Could you check a few things on this model? Use its own coordinates, in mm. Face numbers are marked on the shaded views. A direction names the side the tool comes from. Give positions to 0.01 mm unless a question says otherwise; leave off trailing zeros. Loops run counter-clockwise (first coordinate to the right, second up) from the corner with the lowest first, then second, coordinate; pieces in that order, holes last. Notation, with made-up numbers: (67, -7.75) -> (108, -7.75) arc R14 cw to (108, 8.25) -> close; hole circle Ø11 at (70.25, 79). An arc over 180 degrees is marked (long way). Write item = value, one per line. Start each with the question number.
1) I want a section at C-C (y = 8). Count the separate pieces of the cut face and the enclosed holes in it, and give its area (3 significant figures).
2) If we mould it in two halves opening along Z, with no side actions, what happens to the marked faces 1, 2 and 3? For each: +Z half, -Z half, draft (parallel to the pull), parting line (faces both ways), or undercut.
3) I want a section at D-D (z = -67). List the corners of the cut face in (x, y) for me, and give its area (3 significant figures).
4) I want a section at B-B (z = -5). List the corners of the cut face in (x, y) for me, and give its area (3 significant figures).
5) I'm going to push a flat-ended pin straight in: pin 1 Ø3.5 at (x, z) = (-5, -50.5) entering from +Y. Where does the tip first touch, or does it pass through?
6) On a 3-axis mill with a long thin cutter (end or side, diameter ignored), from which of +Z, -Z, +X, -X, +Y, -Y can I reach the whole of each face in a straight line? I mean the marked faces 4 and 5. Say none if no direction works.
7) I need wall thicknesses on probe 1 along Z at (x, y) = (-5.5, 1.7); probe 2 along Z at (x, y) = (-2.25, 12); probe 3 along Y at (x, z) = (2.75, -76). Which ranges of each line are inside material? Lowest first, please. Write a range as from..to.
8) I want a section at A-A (x = -5.5). List the corners of the cut face in (y, z) for me.
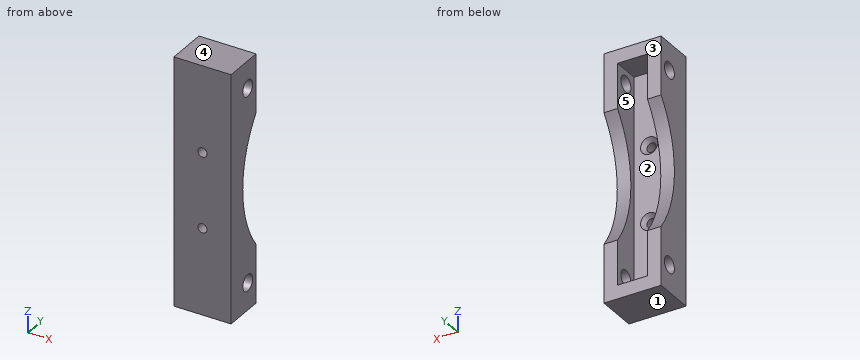
Autodesk Inventor part; units mm, degrees
ref_plane "YZ Plane" through (0, 0, 0) normal (1, 0, 0) x (0, 1, 0)
ref_plane "XZ Plane" through (0, 0, 0) normal (0, 1, 0) x (-1, 0, 0)
ref_plane "XY Plane" through (0, 0, 0) normal (0, 0, 1) x (1, 0, 0)
sketch "Boceto1" plane through (0, 0, 0) normal (0, 1, 0) x (-1, 0, 0)
  point P0 (0, 0)
sketch "Boceto2" plane through (0, 0, 0) normal (0, 1, 0) x (-1, 0, 0)
  line L0 (0, 0) -> (11, 0)
  line L1 (11, 0) -> (11, -81)
  line L2 (11, -81) -> (0, -81)
  line L3 (0, -81) -> (0, 0)
  line L4 (-5, 0) -> (-5, 5)
  line L5 (11, -86) -> (16, -86)
  line L6 (-5, 5) -> (16, 5)
  line L7 (16, 5) -> (16, -86)
  line L8 (16, -86) -> (-5, -86)
  line L9 (-5, -86) -> (-5, 5)
  dimension "d0" = 81
  dimension "d1" = 5
  dimension "d2" = 5
  dimension "d3" = 5
  dimension "d4" = 5
extrude "Extrusión1" add sketch "Boceto2" along normal blind 15
sketch "Boceto3" plane through (0, 0, 0) normal (0, -1, 0) x (1, 0, 0)
  line L0 (0, -81) -> (0, 0)
  line L1 (-11, 0) -> (-11, -81)
  line L2 (0, 0) -> (-11, 0)
  line L3 (-11, 0) -> (-11, -81)
  line L4 (-11, -81) -> (0, -81)
  line L5 (0, -81) -> (0, 0)
extrude "Extrusión2" add sketch "Boceto3" against normal blind 5
sketch "Boceto4" plane through (0, 5, 0) normal (0, 1, 0) x (1, 0, 0)
  line L0 (0, 0) -> (-11, 0)
  line L1 (-5.5, 0) -> (-5.5, 81)
  line L2 (-11, 81) -> (0, 81)
  line L3 (-5.5, 0) -> (-5.5, 26.66)
  line L4 (-5.5, 81) -> (-5.5, 54.34)
  dimension "d9" = 26.66
  dimension "d10" = 26.66
hole "Agujero1" at (-5.5, 5, -26.66) at (-5.5, 5, -54.34) direction (0, -1, 0) diameter 3.4 depth 5 countersink diameter 6.3 countersink angle 90
sketch "Boceto5" plane through (5, 0, 5) normal (1, 0, 0) x (0, 0, -1)
  line L0 (0, 0) -> (45.5, 0)
  line L1 (0, 0) -> (91, 0)
  line L2 (45.5, 0) -> (45.5, 5)
  line L3 (45.5, 5) -> (45.5, 7)
  line L4 (45.5, 7) -> (45.5, 47)
  circle A0 centre (45.5, 47) radius 40
  point P0 (5, 0)
  dimension "d18" = 45.5
  dimension "d19" = 5
  dimension "d20" = 2
  dimension "d21" = 40
extrude "Extrusión3" cut sketch "Boceto5" against normal blind 32
sketch "Boceto6" plane through (5, 0, 5) normal (1, 0, 0) x (0, 0, -1)
  line L0 (0, 0) -> (0, 15)
  line L1 (91, 0) -> (91, 15)
  line L2 (91, 0) -> (0, 0)
  line L3 (0, 0) -> (10, 0)
  line L4 (10, 0) -> (10, 10)
  circle A0 centre (10, 10) radius 3
  line L5 (91, 0) -> (81, 0)
  line L6 (0, 0) -> (91, 0)
  line L7 (81, 0) -> (81, 10)
  circle A1 centre (81, 10) radius 3
  point P0 (5, 0)
  dimension "d26" = 10
  dimension "d27" = 10
  dimension "d29" = 6
  dimension "d30" = 10
  dimension "d31" = 10
sketch "Boceto7" plane through (5, 0, 5) normal (1, 0, 0) x (0, 0, -1)
  line L0 (5, 5) -> (45.5, 5)
  line L1 (86, 5) -> (5, 5)
  point P0 (5, 0)
extrude "Extrusión4" cut sketch "Boceto6" against normal blind 58
properties part number "Base ventilador ahora si"
Answer list:
q1.separate_pieces = 6
q1.enclosed_holes = 0
q1.area = 753 mm^2
q2.face_1 = -Z half
q2.face_2 = undercut
q2.face_3 = draft
q3.outline = (-16, 0) -> (5, 0) -> (5, 15) -> (0, 15) -> (0, 5) -> (-11, 5) -> (-11, 15) -> (-16, 15) -> close
q3.area = 205 mm^2
q4.outline = (-16, 0) -> (5, 0) -> (5, 7) -> (0, 7) -> (0, 5) -> (-11, 5) -> (-11, 7) -> (-16, 7) -> close; (-16, 13) -> (-11, 13) -> (-11, 15) -> (-16, 15) -> close; (0, 13) -> (5, 13) -> (5, 15) -> (0, 15) -> close
q4.area = 145 mm^2
q5.pin_1 = 5
q6.face_4 = +Z, +X, -X, +Y, -Y
q6.face_5 = +Y
q7.probe_1 = -86..-56.04, -52.64..-28.36, -24.96..5
q7.probe_2 = -86..-81, 0..5
q7.probe_3 = 0..7, 13..15
q8.outline = (0, -86) -> (15, -86) -> (15, -81) -> (5, -81) -> (5, -57.49) -> (3.55, -56.04) -> (0, -56.04) -> close; (0, -52.64) -> (3.55, -52.64) -> (5, -51.19) -> (5, -29.81) -> (3.55, -28.36) -> (0, -28.36) -> close; (0, -24.96) -> (3.55, -24.96) -> (5, -23.51) -> (5, 0) -> (15, 0) -> (15, 5) -> (0, 5) -> close
